Answer from the drawing. Dimensions are ordinates in mm from the lowest x, y and z of the part. Give positions to 0.01 mm unless a question says otherwise; leave off trailing zeros. Write each loop counter-clockwise with the first axis right and the second up, starting at its lowest first coordinate (ties: lowest second). Pieces come first, ordered by that corner, then holes.
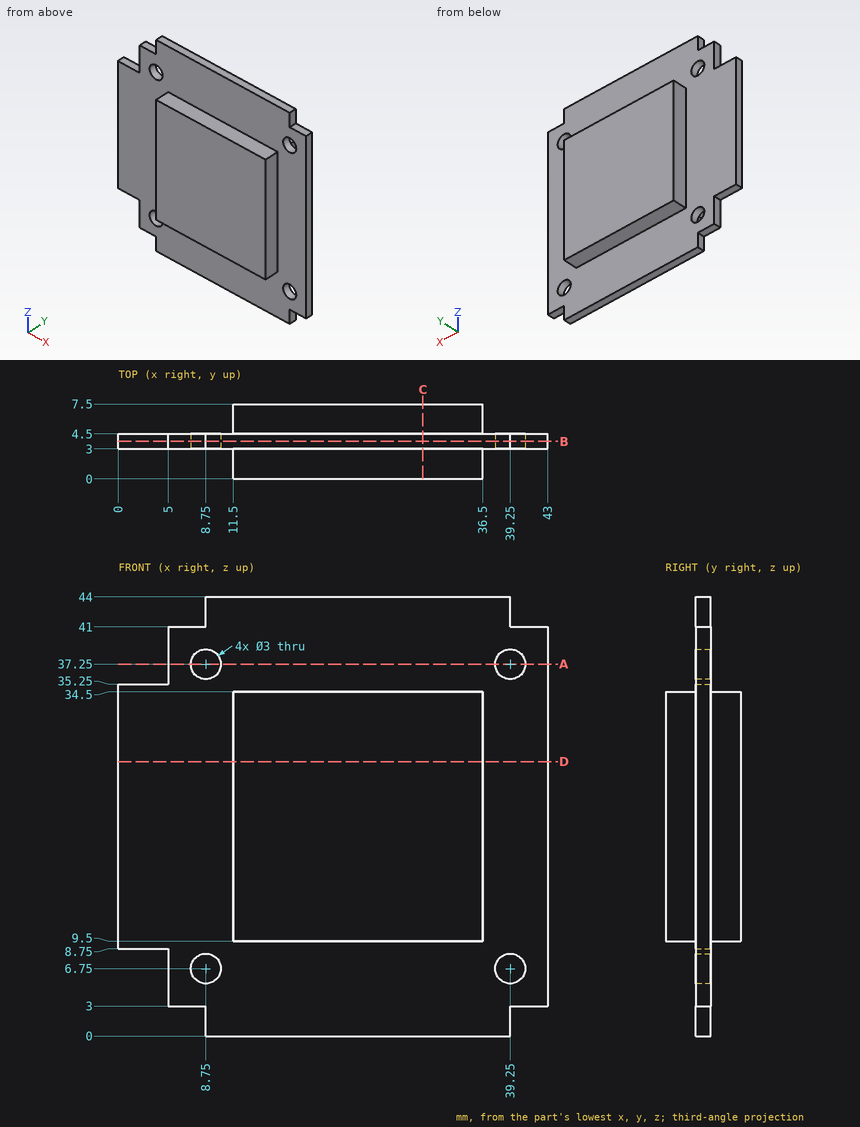
Item 1: A cutting plane is placed at C-C, the plane x = 30.5. Give the vertices of the cut face in (y, z), plus the area to 3 significant figures.
Conclusion:
outline: (0, 9.5) - (3, 9.5) - (3, 0) - (4.5, 0) - (4.5, 9.5) - (7.5, 9.5) - (7.5, 34.5) - (4.5, 34.5) - (4.5, 44) - (3, 44) - (3, 34.5) - (0, 34.5) - close
area: 216 mm2
Item 2: Each of these flat-tipped pins is pushed along its axis until it touches: P1, Ø1.5, axis at x = 20.5, y = 2, coming from the +Z side; P2, Ø0.9, axis at x = 29, y = 1, coming from the -Z side; P3, Ø1.6, axis at x = 3, y = 3.5, coming from the -Z side; P4, Ø1.5, axis at y = 6, z = 7, coming from the -X side. Where does it stop, or does it pass through?
Conclusion:
P1: stops at z = 34.5
P2: stops at z = 9.5
P3: stops at z = 8.75
P4: passes through
Item 3: A cutting plane is placed at B-B, the plane y = 3.75. Give the vertices of the cut face in (x, z).
Conclusion:
outline: (0, 8.75) - (5, 8.75) - (5, 3) - (8.75, 3) - (8.75, 0) - (39.25, 0) - (39.25, 3) - (43, 3) - (43, 41) - (39.25, 41) - (39.25, 44) - (8.75, 44) - (8.75, 41) - (5, 41) - (5, 35.25) - (0, 35.25) - close; hole circle Ø3 at (8.75, 6.75); hole circle Ø3 at (8.75, 37.25); hole circle Ø3 at (39.25, 6.75); hole circle Ø3 at (39.25, 37.25)
Item 4: Consider probe 1 along X at (y, z) = (3.7, 37.25); probe 2 along Z at (x, y) = (7.5, 4); probe 3 along Y at (x, z) = (10.5, 40.5). Determine where each line is inside the solid, lowest interval first.
Conclusion:
probe 1: x = 5 to 7.25, 10.25 to 37.75, 40.75 to 43
probe 2: z = 3 to 5.92, 7.58 to 36.42, 38.08 to 41
probe 3: y = 3 to 4.5
Item 5: A cutting plane is placed at A-A, the plane z = 37.25. Give the vertices of the cut face in (x, y), plus the area to 3 significant figures.
Conclusion:
outline: (5, 3) - (7.25, 3) - (7.25, 4.5) - (5, 4.5) - close; (10.25, 3) - (37.75, 3) - (37.75, 4.5) - (10.25, 4.5) - close; (40.75, 3) - (43, 3) - (43, 4.5) - (40.75, 4.5) - close
area: 48.0 mm2
Item 6: A cutting plane is placed at D-D, the plane z = 27.5. Give the vertices of the cut face in (x, y), plus the area to 4 significant figures.
Conclusion:
outline: (0, 3) - (11.5, 3) - (11.5, 0) - (36.5, 0) - (36.5, 3) - (43, 3) - (43, 4.5) - (36.5, 4.5) - (36.5, 7.5) - (11.5, 7.5) - (11.5, 4.5) - (0, 4.5) - close
area: 214.5 mm2
